from build123d import *

# Parameters (mm, degrees)
SKETCH1_W            = 80
SKETCH1_H            = 20
SKETCH1_R            = 2
BOSS_EXTRUDE1_DEPTH  = 5
BOSS_EXTRUDE2_DEPTH  = 5
BOSS_EXTRUDE3_DEPTH  = 5
BOSS_EXTRUDE4_DEPTH  = 5
BOSS_EXTRUDE9_DEPTH  = 5
BOSS_EXTRUDE10_DEPTH = 5


with BuildPart() as part:
    # Sketch1 → Boss-Extrude1 (new body)
    with BuildSketch(Plane.XY):
        with Locations((0.15936255, 5.458167331)):
            Rectangle(SKETCH1_W, SKETCH1_H)
        with Locations((-29.84063745, 5.458167331)):
            Circle(SKETCH1_R, mode=Mode.SUBTRACT)
        with Locations((30.15936255, 5.458167331)):
            Circle(SKETCH1_R, mode=Mode.SUBTRACT)
    extrude(amount=BOSS_EXTRUDE1_DEPTH)

    # Sketch2 → Boss-Extrude2 (add)
    with BuildSketch(Plane(origin=(12, 0, 0), x_dir=(0, 0, -1), z_dir=(1, 0, 0))):
        Polygon((0, 15.458167331), (21.213203436, -5.755036105), (21.213203436, -25.755036105), (0, -4.541832669), align=None)
    extrude(amount=BOSS_EXTRUDE2_DEPTH)

    # Sketch3 → Boss-Extrude3 (add)
    with BuildSketch(Plane(origin=(-12, 0, 0), x_dir=(0, 0, -1), z_dir=(1, 0, 0))):
        Polygon((0, 15.458167331), (21.213203436, -5.755036105), (21.213203436, -25.755036105), (0, -4.541832669), align=None)
    extrude(amount=-BOSS_EXTRUDE3_DEPTH)

    # Sketch4 → Boss-Extrude4 (add)
    with BuildSketch(Plane(origin=(0, 0, -21.213203436), x_dir=(-1, 0, 0), z_dir=(0, 0, -1))):
        Polygon((65, -5.755036105), (-17, -5.755036105), (-65, -5.755036105), (-65, -25.127384199), (-65, -32.826103917), (-65, -35.755036105), (65, -35.755036105), (65, -32.826103917), (65, -25.561464244), align=None)
    extrude(amount=BOSS_EXTRUDE4_DEPTH)

    # Sketch6 → Boss-Extrude9 (add)
    with BuildSketch(Plane(origin=(63, 0, 0), x_dir=(0, 0, -1), z_dir=(1, 0, 0))):
        Polygon((26.213203436, -5.755036105), (33.941125497, -13.482958166), (33.941125497, -50.554025978), (33.941125497, -55.554025978), (33.941125497, -57.482958166), (21.213203436, -44.755036105), (19.798989873, -43.340822543), (19.798989873, 0.659177457), (21.213203436, -0.755036105), align=None)
    extrude(amount=BOSS_EXTRUDE9_DEPTH)

    # Sketch8 → Boss-Extrude10 (add)
    with BuildSketch(Plane.ZY.offset(63)):
        Polygon((-19.798989873, 0.659177457), (-33.941125497, -13.482958166), (-33.941125497, -57.482958166), (-19.798989873, -43.340822543), align=None)
    extrude(amount=BOSS_EXTRUDE10_DEPTH)


solid = part.part
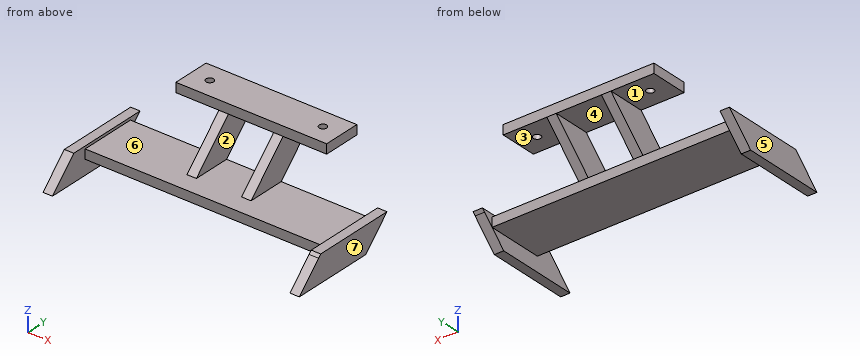
Read the model definition and answer for the solid it produces. Units are mm, in the model's axes. Face numbers are marked on the shaded views. A direction names the side the tool comes from. Coordinates: 2 decimals unless noted, no trailing zeros. Write each loop counter-clockwise with the first axis right and the second up, starting at its lowest first coordinate (ties: lowest second). Pieces come first, ordered by that corner, then holes. Notation, with made-up numbers: (68, 26) -> (118, 26) arc R25 cw to (118, 61) -> close; hole circle Ø7 at (43, 30). An arc over 180 degrees is marked (long way). Return JSON: item names as keys, results as strings.
(1) The part is cut by section D-D on z = 2.5. Give the vertices of the cut face in (x, y), then the cut area to 3 significant figures.
Answers below:
{"outline": "(-39.84, -4.54) -> (40.16, -4.54) -> (40.16, 15.46) -> (-39.84, 15.46) -> close; hole circle Ø4 at (-29.84, 5.46); hole circle Ø4 at (30.16, 5.46)", "area": "1,570 mm^2"}
(2) Each of these flat-tipped pins is pushed along its axis until it touches: P1, Ø3, axis at x = 26, y = -19.5, coming from the -Z side; P2, Ø8, axis at y = -22.5, z = -7, coming from the -X side; P3, Ø6, axis at x = 24, y = 10, coming from the -Z side; P4, Ø2.5, axis at x = 64.5, y = -25.5, coming from the +Z side. Where does it stop, or does it pass through?
Answers below:
{"P1": "z = -26.21", "P2": "through", "P3": "z = 0", "P4": "z = -19.8"}
(3) The part is cut by section A-A on x = 24.5. Give the vertices of the cut face in (y, z), then the cut area to 3 significant figures.
Answers below:
{"outline": "(-35.76, -26.21) -> (-5.76, -26.21) -> (-5.76, -21.21) -> (-35.76, -21.21) -> close; (-4.54, 0) -> (15.46, 0) -> (15.46, 5) -> (-4.54, 5) -> close", "area": "250 mm^2"}
(4) The part is cut by section B-B on y = -40. Give the vertices of the cut face in (x, z).
Answers below:
{"outline": "(-68, -33.94) -> (-63, -33.94) -> (-63, -19.8) -> (-68, -19.8) -> close; (63, -33.94) -> (68, -33.94) -> (68, -19.8) -> (63, -19.8) -> close"}
(5) The part is cut by section C-C on y = -30. Give the vertices of the cut face in (x, z).
Answers below:
{"outline": "(-68, -33.94) -> (-63, -33.94) -> (-63, -26.21) -> (63, -26.21) -> (63, -33.94) -> (68, -33.94) -> (68, -19.8) -> (63, -19.8) -> (63, -21.21) -> (-63, -21.21) -> (-63, -19.8) -> (-68, -19.8) -> close"}
(6) Consider line 1 along X through (y, z) = (-37, -26); line 2 along Z through (x, y) = (54.5, -20); line 3 along Y through (x, z) = (23.5, 2). Determine where each line is inside the solid, lowest interval first. Write a range as from..to.
Answers below:
{"line 1": "-68..-63, 63..68", "line 2": "-26.21..-21.21", "line 3": "-4.54..15.46"}
(7) Which of the six approach directions +Z, -Z, +X, -X, +Y, -Y give full straight-line access (tool end or side, diameter ignored) to the marked faces 1, 2, 3 and 4?
Answers below:
{"face 1": "-Z, -X, +Y, -Y", "face 2": "+Y, -Y", "face 3": "-Z, +X, +Y, -Y", "face 4": "-Z, +Y, -Y"}
(8) For a pull along X with two mould halves and no side action, classify the marked faces 5, 6 and 7 as pulls with the +X half, pulls with the -X half, needs draft (parallel to the pull), parting line crosses it, or undercut.
Answers below:
{"face 5": "pulls with the -X half", "face 6": "undercut", "face 7": "pulls with the +X half"}
